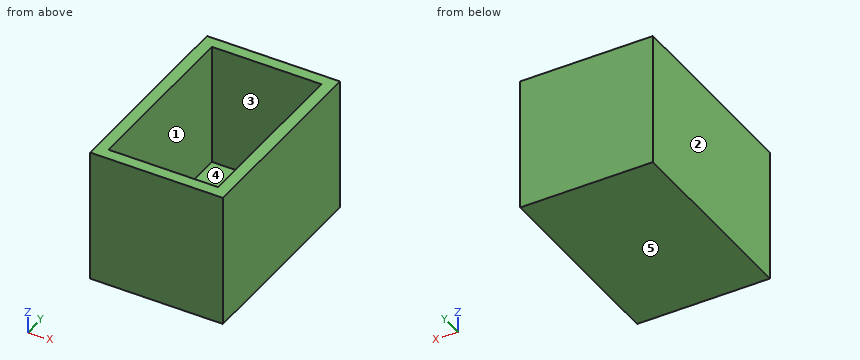
from build123d import *

# Parameters (mm, degrees)
F1_W     = 28.9652645588
F1_H     = 43.5288026929
F2_DEPTH = 3.81
F3_DEPTH = 25.4
F4_T     = -2.54


# Not quite as in the source:
# - a feature of the source that left no trace in its solid (it failed there, or was rolled back) is left out


with BuildPart() as f2:
    # F1 (on Top) → F2 (new body)
    with BuildSketch(Plane.XY):
        with Locations((29.5196138322, -1.5338174999)):
            Rectangle(F1_W, F1_H)
    extrude(amount=F2_DEPTH)

    # F3 (add): a face of the model
    f3_faces = [f2.faces().sort_by_distance(p)[0] for p in [
        (29.5196138322, -1.5338174999, 3.81),
    ]]
    extrude(f3_faces, amount=F3_DEPTH)

    # F4
    f4_openings = [f2.faces().sort_by_distance(p)[0] for p in [
        (29.519614, -1.533817, 29.21),
    ]]
    offset(amount=F4_T, openings=f4_openings)


solid = f2.part
Geometry: final body of the model. Coordinates: model frame, mm. Face numbers are marked on the shaded views. A direction names the side the tool comes from. Coordinates: 2 decimals unless noted, no trailing zeros. Order: outer loops, then holes, each group sorted by start corner. A loop starts at its lowest first (then second) coordinate and runs counter-clockwise, first axis right, second up.
(1) Material intervals for probe 1 along Y at (x, z) = (24.25, 12.25); probe 2 along X at (y, z) = (-1, 21.75); probe 3 along Z at (x, y) = (20, -18.5), sorted ascending.
(2) Section query C-C (y = -3.5). Return the cut outline in (x, z), plus the area to 3 significant figures.
(3) Section query B-B (z = 20). Return the cut outline in (x, y), plus the area to 3 significant figures.
(4) First-contact query: pin 1 (3 mm diameter, centred on x = 26.5, y = 12, fed in from +Z). Flat tip, straight axial feed; report the tip coordinate or a pass-through.
(5) Access query for the marked faces 1 and 2. Directions: +Z, -Z, +X, -X, +Y, -Y. A direction counts if a zero-diameter tool reaches every point of the face in a straight line with its end or side. Return the directions, or none.
(6) Draft query along Z for the marked faces 3, 4 and 5. Return one class per face: pulls with the +Z half, pulls with the -Z half, needs draft (parallel to the pull), parting line crosses it, or undercut.
(7) Section query A-A (x = 37.5). Return the cut outline in (y, z).
Solution:
1. probe 1: y = -23.3 to -20.76, 17.69 to 20.23
1. probe 2: x = 15.04 to 17.58, 41.46 to 44
1. probe 3: z = 0 to 2.54
2. outline: (15.04, 0) - (44, 0) - (44, 29.21) - (41.46, 29.21) - (41.46, 2.54) - (17.58, 2.54) - (17.58, 29.21) - (15.04, 29.21) - close
2. area: 209 mm2
3. outline: (15.04, -23.3) - (44, -23.3) - (44, 20.23) - (15.04, 20.23) - close; hole (17.58, -20.76) - (41.46, -20.76) - (41.46, 17.69) - (17.58, 17.69) - close
3. area: 342 mm2
4. pin 1: stops at z = 2.54
5. face 1: +Z
5. face 2: +Z, -Z, -X, +Y, -Y
6. face 3: needs draft
6. face 4: pulls with the +Z half
6. face 5: pulls with the -Z half
7. outline: (-23.3, 0) - (20.23, 0) - (20.23, 29.21) - (17.69, 29.21) - (17.69, 2.54) - (-20.76, 2.54) - (-20.76, 29.21) - (-23.3, 29.21) - close
